The model under review builds one solid part; all positions refer to its coordinate system, in mm. A direction names the side the tool comes from. Round coordinates to 2 decimals unless told otherwise and drop trailing zeros. Order: outer loops, then holes, each group sorted by start corner. A loop starts at its lowest first (then second) coordinate and runs counter-clockwise, first axis right, second up.
1) Consider section A-A (z = -12.5). Give the boundary of the cut face in (x, y), then the cut area to 3 significant figures.
2) Clearance check with flat-ended pins moving along their axes: P1, Ø0.8, axis at x = 2, z = 1, coming from the +Y side; P2, Ø1.4, axis at x = 1, z = 7.5, coming from the -Y side; P3, Ø3.5, axis at y = -7, z = -11.5, coming from the +X side; P4, Ø1.5, axis at x = 4, y = 7, coming from the +Z side. State where each tip first meets the part, or that it passes through.
3) Machinability: for faces 1 (the face through (1.609, -2.559, 26.606)), 2 (the face through (1, -2.921, 0)), 3 (the face through (2.794, 5, 0)), 4 (the face through (3.18, 3.97, -26.63)), 5 (the face through (1.609, -2.539, -26.625)), which of the approach directions +Z, -Z, +X, -X, +Y, -Y give a long, thin tool a straight path to every point of the face, cutting with its end or side? Answer none if there is none.
4) Consider section B-B (x = 1.5). Give the boundary of the cut face in (y, z), then the cut area to 3 significant figures.
5) To check wall thickness, follow L1, parallel to X at y = -9.5, z = -1; L2, parallel to Y at x = 2.5, z = -8; L3, parallel to Y at x = 3, z = 24.5. State the ranges of each line that lie inside material, in increasing order.
6) Consider section C-C (y = 11.5). Give the boundary of the cut face in (x, z), then the cut area to 3 significant figures.
from build123d import *

# Parameters (mm, degrees)
BOSS_EXTRUDE1_DEPTH = 53.975
SKETCH2_W           = 6.858
SKETCH2_H           = 3.429
CUT_EXTRUDE1_DEPTH  = 55.91468839
SKETCH4_W           = 6.858
SKETCH4_H           = 3.429
CUT_EXTRUDE2_DEPTH  = 55.91468839
SKETCH18_W          = 53.975
SKETCH18_H          = 26.924
BOSS_EXTRUDE5_DEPTH = 4.064
FILLET1_R           = 1.27
FILLET3_R           = 1.27
FILLET5_R           = 1.27


with BuildPart() as part:
    # Sketch1 → Boss-Extrude1 (new body)
    with BuildSketch(Plane.XY.offset(26.9875)):
        Polygon((3.302, 6.35), (-4.064, 6.35), (-4.064, -6.35), (3.302, -6.35), (7.874, -2.54), (7.874, 2.54), align=None)
    extrude(amount=-BOSS_EXTRUDE1_DEPTH)

    # Sketch2 → Cut-Extrude1 (cut, through all)
    with BuildSketch(Plane.XY.offset(26.9875)):
        with Locations((-0.635, 4.6355)):
            Rectangle(SKETCH2_W, SKETCH2_H)
    extrude(amount=-CUT_EXTRUDE1_DEPTH, mode=Mode.SUBTRACT)

    # Sketch4 → Cut-Extrude2 (cut, through all)
    with BuildSketch(Plane.XY.offset(26.9875)):
        with Locations((-0.635, -4.6355)):
            Rectangle(SKETCH4_W, SKETCH4_H)
    extrude(amount=-CUT_EXTRUDE2_DEPTH, mode=Mode.SUBTRACT)

    # Sketch18 → Boss-Extrude5 (add)
    with BuildSketch(Plane.ZY.offset(4.064)):
        Rectangle(SKETCH18_W, SKETCH18_H)
    extrude(amount=-BOSS_EXTRUDE5_DEPTH)

    # Fillet1
    fillet1_edges = [part.edges().sort_by_distance(p)[0] for p in [
        (7.874, 2.54, 0),
        (7.874, -2.54, 0),
    ]]
    fillet(fillet1_edges, radius=FILLET1_R)

    # Fillet3
    # the kernel refuses this fillet: 1.27 mm, written as the material it takes off along each edge
    with BuildSketch(Plane(origin=(0.862897437, -8.382585469, -26.9875), x_dir=(-0.6401843996644798, 0.7682212795973759, 0), z_dir=(0.7682212795973759, 0.6401843996644799, 0))) as fillet3_piece_1:
        with BuildLine():
            CenterArc((FILLET3_R, FILLET3_R), FILLET3_R, 180, 90)
            Line((0, FILLET3_R), (0, 0))
            Line((0, 0), (FILLET3_R, 0))
        make_face()
    extrude(amount=8.531574072, mode=Mode.SUBTRACT)
    with BuildSketch(Plane(origin=(6.604, -1.945163819, -26.9875), x_dir=(1, 0, 0), z_dir=(0, 1, 0))) as fillet3_piece_2:
        with BuildLine():
            CenterArc((1.27 - FILLET3_R, -FILLET3_R), FILLET3_R, 0, 90)
            Line((1.27, -FILLET3_R), (1.27, 0))
            Line((1.27, 0), (1.27 - FILLET3_R, 0))
        make_face()
    revolve(axis=Axis((6.604, -1.945163819, -26.9875), (0, 0, -1)), revolution_arc=50.194428908, mode=Mode.SUBTRACT)
    with BuildSketch(Plane(origin=(7.417034188, 2.920804844, -26.9875), x_dir=(0, 0, 1), z_dir=(-0.7682212795973759, 0.6401843996644799, 0))) as fillet3_piece_3:
        with BuildLine():
            CenterArc((FILLET3_R, -FILLET3_R), FILLET3_R, 90, 90)
            Line((0, -FILLET3_R), (0, 0))
            Line((0, 0), (FILLET3_R, 0))
        make_face()
    extrude(amount=8.531574072, mode=Mode.SUBTRACT)
    with BuildSketch(Plane(origin=(6.604, 1.945163819, -26.9875), x_dir=(0.6401843996644799, 0.7682212795973757, 0), z_dir=(-0.7682212795973757, 0.6401843996644799, 0))) as fillet3_piece_4:
        with BuildLine():
            CenterArc((1.27 - FILLET3_R, -FILLET3_R), FILLET3_R, 0, 90)
            Line((1.27 - FILLET3_R, 0), (1.27, 0))
            Line((1.27, 0), (1.27, -FILLET3_R))
        make_face()
    revolve(axis=Axis((6.604, 1.945163819, -26.9875), (0, 0, -1)), revolution_arc=50.194428908, mode=Mode.SUBTRACT)
    with BuildSketch(Plane(origin=(2.794, -2.921, -26.9875), x_dir=(0, 1, 0), z_dir=(-1, 0, 0)), Plane(origin=(0, 2.921, -26.9875), x_dir=(0, -1, 0), z_dir=(1, 0, 0))) as fillet3_piece_5:
        with BuildLine():
            CenterArc((FILLET3_R, -FILLET3_R), FILLET3_R, 90, 90)
            Line((0, -FILLET3_R), (0, 0))
            Line((0, 0), (FILLET3_R, 0))
        make_face()
    extrude(amount=2.794, mode=Mode.SUBTRACT)
    with BuildSketch(Plane(origin=(2.794, 2.921, -26.9875), x_dir=(1, 0, 0), z_dir=(0, 1, 0)), Plane(origin=(2.794, -9.525, -26.9875), x_dir=(1, 0, 0), z_dir=(0, 1, 0))) as fillet3_piece_6:
        with BuildLine():
            CenterArc((FILLET3_R, -FILLET3_R), FILLET3_R, 90, 90)
            Line((0, -FILLET3_R), (0, 0))
            Line((0, 0), (FILLET3_R, 0))
        make_face()
    extrude(amount=6.604, mode=Mode.SUBTRACT)
    with BuildSketch(Plane(origin=(7.874, -1.945163819, -26.9875), x_dir=(-1, 0, 0), z_dir=(0, 1, 0))) as fillet3_piece_7:
        with BuildLine():
            CenterArc((FILLET3_R, FILLET3_R), FILLET3_R, 180, 90)
            Line((0, FILLET3_R), (0, 0))
            Line((0, 0), (FILLET3_R, 0))
        make_face()
    extrude(amount=3.890327637, mode=Mode.SUBTRACT)
    with BuildSketch(Plane(origin=(2.794, -9.525, -26.9875), x_dir=(1, 0, 0), z_dir=(0, 1, 0))) as fillet3_piece_8a_section:
        with BuildLine():
            CenterArc((FILLET3_R, -FILLET3_R), FILLET3_R, 90, 90)
            Line((0, -FILLET3_R), (0, 0))
            Line((0, 0), (FILLET3_R, 0))
        make_face()
    fillet3_piece_8a = extrude(amount=9.779, mode=Mode.PRIVATE)
    fillet3_piece_8a = split(fillet3_piece_8a, bisect_by=Plane(origin=(3.081521795, -2.921, -26.699978205), z_dir=(0, 1, 0)), keep=Keep.TOP, mode=Mode.PRIVATE)
    with BuildSketch(Plane(origin=(5.969, -2.921, -26.9875), x_dir=(0, 1, 0), z_dir=(-1, 0, 0))) as fillet3_piece_8b_section:
        with BuildLine():
            CenterArc((FILLET3_R, -FILLET3_R), FILLET3_R, 90, 90)
            Line((0, -FILLET3_R), (0, 0))
            Line((0, 0), (FILLET3_R, 0))
        make_face()
    fillet3_piece_8b = extrude(amount=5.969, mode=Mode.PRIVATE)
    fillet3_piece_8b = split(fillet3_piece_8b, bisect_by=Plane(origin=(2.794, -2.633478205, -26.699978205), z_dir=(1, 0, 0)), keep=Keep.TOP, mode=Mode.PRIVATE)
    fillet3_piece_8 = fillet3_piece_8a & fillet3_piece_8b
    add(fillet3_piece_8, mode=Mode.SUBTRACT)
    with BuildSketch(Plane(origin=(2.794, -0.254, -26.9875), x_dir=(1, 0, 0), z_dir=(0, 1, 0))) as fillet3_piece_9a_section:
        with BuildLine():
            CenterArc((FILLET3_R, -FILLET3_R), FILLET3_R, 90, 90)
            Line((0, -FILLET3_R), (0, 0))
            Line((0, 0), (FILLET3_R, 0))
        make_face()
    fillet3_piece_9a = extrude(amount=9.779, mode=Mode.PRIVATE)
    fillet3_piece_9a = split(fillet3_piece_9a, bisect_by=Plane(origin=(3.081521795, 2.921, -26.699978205), z_dir=(0, -1, 0)), keep=Keep.TOP, mode=Mode.PRIVATE)
    with BuildSketch(Plane(origin=(0, 2.921, -26.9875), x_dir=(0, -1, 0), z_dir=(1, 0, 0))) as fillet3_piece_9b_section:
        with BuildLine():
            CenterArc((FILLET3_R, -FILLET3_R), FILLET3_R, 90, 90)
            Line((0, -FILLET3_R), (0, 0))
            Line((0, 0), (FILLET3_R, 0))
        make_face()
    fillet3_piece_9b = extrude(amount=5.969, mode=Mode.PRIVATE)
    fillet3_piece_9b = split(fillet3_piece_9b, bisect_by=Plane(origin=(2.794, 2.633478205, -26.699978205), z_dir=(1, 0, 0)), keep=Keep.TOP, mode=Mode.PRIVATE)
    fillet3_piece_9 = fillet3_piece_9a & fillet3_piece_9b
    add(fillet3_piece_9, mode=Mode.SUBTRACT)

    # Fillet5
    # the kernel refuses this fillet: 1.27 mm, written as the material it takes off along each edge
    with BuildSketch(Plane(origin=(0.862897437, -8.382585469, 26.9875), x_dir=(0, 0, -1), z_dir=(0.7682212795973759, 0.6401843996644799, 0)), Plane(origin=(7.417034188, 2.920804844, 26.9875), x_dir=(0, 0, -1), z_dir=(-0.7682212795973759, 0.6401843996644799, 0))) as fillet5_piece_1:
        with BuildLine():
            CenterArc((FILLET5_R, FILLET5_R), FILLET5_R, 180, 90)
            Line((0, FILLET5_R), (0, 0))
            Line((0, 0), (FILLET5_R, 0))
        make_face()
    extrude(amount=8.531574072, mode=Mode.SUBTRACT)
    with BuildSketch(Plane(origin=(6.604, -1.945163819, 26.9875), x_dir=(1, 0, 0), z_dir=(0, 1, 0))) as fillet5_piece_2:
        with BuildLine():
            CenterArc((1.27 - FILLET5_R, FILLET5_R), FILLET5_R, 270, 90)
            Line((1.27 - FILLET5_R, 0), (1.27, 0))
            Line((1.27, 0), (1.27, FILLET5_R))
        make_face()
    revolve(axis=Axis((6.604, -1.945163819, 26.9875), (0, 0, -1)), revolution_arc=50.194428908, mode=Mode.SUBTRACT)
    with BuildSketch(Plane(origin=(6.604, 1.945163819, 26.9875), x_dir=(0.6401843996644799, 0.7682212795973757, 0), z_dir=(-0.7682212795973757, 0.6401843996644799, 0))) as fillet5_piece_3:
        with BuildLine():
            CenterArc((1.27 - FILLET5_R, FILLET5_R), FILLET5_R, 270, 90)
            Line((1.27 - FILLET5_R, 0), (1.27, 0))
            Line((1.27, 0), (1.27, FILLET5_R))
        make_face()
    revolve(axis=Axis((6.604, 1.945163819, 26.9875), (0, 0, -1)), revolution_arc=50.194428908, mode=Mode.SUBTRACT)
    with BuildSketch(Plane(origin=(2.794, 2.921, 26.9875), x_dir=(0, 0, -1), z_dir=(0, 1, 0)), Plane(origin=(2.794, -9.525, 26.9875), x_dir=(0, 0, -1), z_dir=(0, 1, 0))) as fillet5_piece_4:
        with BuildLine():
            CenterArc((FILLET5_R, -FILLET5_R), FILLET5_R, 90, 90)
            Line((0, -FILLET5_R), (0, 0))
            Line((0, 0), (FILLET5_R, 0))
        make_face()
    extrude(amount=6.604, mode=Mode.SUBTRACT)
    with BuildSketch(Plane(origin=(0, 2.921, 26.9875), x_dir=(0, 0, -1), z_dir=(1, 0, 0)), Plane(origin=(2.794, -2.921, 26.9875), x_dir=(0, 0, -1), z_dir=(-1, 0, 0))) as fillet5_piece_5:
        with BuildLine():
            CenterArc((FILLET5_R, -FILLET5_R), FILLET5_R, 90, 90)
            Line((0, -FILLET5_R), (0, 0))
            Line((0, 0), (FILLET5_R, 0))
        make_face()
    extrude(amount=2.794, mode=Mode.SUBTRACT)
    with BuildSketch(Plane(origin=(7.874, -1.945163819, 26.9875), x_dir=(0, 0, -1), z_dir=(0, 1, 0))) as fillet5_piece_6:
        with BuildLine():
            CenterArc((FILLET5_R, FILLET5_R), FILLET5_R, 180, 90)
            Line((0, FILLET5_R), (0, 0))
            Line((0, 0), (FILLET5_R, 0))
        make_face()
    extrude(amount=3.890327637, mode=Mode.SUBTRACT)
    with BuildSketch(Plane(origin=(0, 2.921, 26.9875), x_dir=(0, 0, -1), z_dir=(1, 0, 0))) as fillet5_piece_7a_section:
        with BuildLine():
            CenterArc((FILLET5_R, -FILLET5_R), FILLET5_R, 90, 90)
            Line((0, -FILLET5_R), (0, 0))
            Line((0, 0), (FILLET5_R, 0))
        make_face()
    fillet5_piece_7a = extrude(amount=5.969, mode=Mode.PRIVATE)
    fillet5_piece_7a = split(fillet5_piece_7a, bisect_by=Plane(origin=(2.794, 2.633478205, 26.699978205), z_dir=(1, 0, 0)), keep=Keep.TOP, mode=Mode.PRIVATE)
    with BuildSketch(Plane(origin=(2.794, -0.254, 26.9875), x_dir=(0, 0, -1), z_dir=(0, 1, 0))) as fillet5_piece_7b_section:
        with BuildLine():
            CenterArc((FILLET5_R, -FILLET5_R), FILLET5_R, 90, 90)
            Line((0, -FILLET5_R), (0, 0))
            Line((0, 0), (FILLET5_R, 0))
        make_face()
    fillet5_piece_7b = extrude(amount=9.779, mode=Mode.PRIVATE)
    fillet5_piece_7b = split(fillet5_piece_7b, bisect_by=Plane(origin=(3.081521795, 2.921, 26.699978205), z_dir=(0, -1, 0)), keep=Keep.TOP, mode=Mode.PRIVATE)
    fillet5_piece_7 = fillet5_piece_7a & fillet5_piece_7b
    add(fillet5_piece_7, mode=Mode.SUBTRACT)
    with BuildSketch(Plane(origin=(2.794, -9.525, 26.9875), x_dir=(0, 0, -1), z_dir=(0, 1, 0))) as fillet5_piece_8a_section:
        with BuildLine():
            CenterArc((FILLET5_R, -FILLET5_R), FILLET5_R, 90, 90)
            Line((0, -FILLET5_R), (0, 0))
            Line((0, 0), (FILLET5_R, 0))
        make_face()
    fillet5_piece_8a = extrude(amount=9.779, mode=Mode.PRIVATE)
    fillet5_piece_8a = split(fillet5_piece_8a, bisect_by=Plane(origin=(3.081521795, -2.921, 26.699978205), z_dir=(0, 1, 0)), keep=Keep.TOP, mode=Mode.PRIVATE)
    with BuildSketch(Plane(origin=(5.969, -2.921, 26.9875), x_dir=(0, 0, -1), z_dir=(-1, 0, 0))) as fillet5_piece_8b_section:
        with BuildLine():
            CenterArc((FILLET5_R, -FILLET5_R), FILLET5_R, 90, 90)
            Line((0, -FILLET5_R), (0, 0))
            Line((0, 0), (FILLET5_R, 0))
        make_face()
    fillet5_piece_8b = extrude(amount=5.969, mode=Mode.PRIVATE)
    fillet5_piece_8b = split(fillet5_piece_8b, bisect_by=Plane(origin=(2.794, -2.633478205, 26.699978205), z_dir=(1, 0, 0)), keep=Keep.TOP, mode=Mode.PRIVATE)
    fillet5_piece_8 = fillet5_piece_8a & fillet5_piece_8b
    add(fillet5_piece_8, mode=Mode.SUBTRACT)


solid = part.part
Answer below:
1. outline: (-4.06, -13.46) - (0, -13.46) - (0, -2.92) - (2.79, -2.92) - (2.79, -6.35) - (3.3, -6.35) - (7.42, -2.92) arc R1.27 ccw to (7.87, -1.95) - (7.87, 1.95) arc R1.27 ccw to (7.42, 2.92) - (3.3, 6.35) - (2.79, 6.35) - (2.79, 2.92) - (0, 2.92) - (0, 13.46) - (-4.06, 13.46) - close
1. area: 173 mm2
2. P1: stops at y = 2.92
2. P2: stops at y = -2.92
2. P3: stops at x = 4.62
2. P4: passes through
3. face 1: +Z, -Y
3. face 2: +Z, -Z, -Y
3. face 3: +Z, -Z, +Y
3. face 4: -Z, +Y
3. face 5: -Z, -Y
4. outline: (-2.92, -25.72) arc R1.27 ccw to (-1.65, -26.99) - (1.65, -26.99) arc R1.27 ccw to (2.92, -25.72) - (2.92, 25.72) arc R1.27 ccw to (1.65, 26.99) - (-1.65, 26.99) arc R1.27 ccw to (-2.92, 25.72) - close
4. area: 314 mm2
5. L1: x = -4.06 to 0
5. L2: y = -2.92 to 2.92
5. L3: y = -6.35 to 6.35
6. outline: (-4.06, -26.99) - (0, -26.99) - (0, 26.99) - (-4.06, 26.99) - close
6. area: 219 mm2
